Input: part model. Units: mm. Frame: model coordinates. A direction names the side the tool comes from. Coordinates: 2 decimals unless noted, no trailing zeros. Order: outer loops, then holes, each group sorted by start corner. A loop starts at its lowest first (then second) coordinate and runs counter-clockwise, first axis right, second up. Notation, with made-up numbers: (23, 22) -> (60, 22) arc R19 ccw to (60, 31) -> close; hole circle Ø7 at (-16, -31.75). An arc over 180 degrees is marked (long way). One line per item, written item: value. Start each with the question number.
from build123d import *

# Parameters (mm, degrees)
SKETCH2_W           = 10
SKETCH2_H           = 50
BOSS_EXTRUDE1_DEPTH = 10
SKETCH6_R           = 2.35
CUT_EXTRUDE3_DEPTH  = 11
SKETCH7_R           = 2.35
CUT_EXTRUDE4_DEPTH  = 11
SKETCH8_W           = 1.5
SKETCH8_H           = 21
BOSS_EXTRUDE2_DEPTH = 30


with BuildPart() as part:
    # Sketch2 → Boss-Extrude1 (new body)
    with BuildSketch(Plane.XY):
        with Locations((5, 25)):
            Rectangle(SKETCH2_W, SKETCH2_H)
    extrude(amount=BOSS_EXTRUDE1_DEPTH)

    # Sketch6 → Cut-Extrude3 (cut, through all)
    with BuildSketch(Plane.XY.offset(10)):
        with Locations((5, 27)):
            Circle(SKETCH6_R)
    extrude(amount=-CUT_EXTRUDE3_DEPTH, mode=Mode.SUBTRACT)

    # Sketch7 → Cut-Extrude4 (cut, through all)
    with BuildSketch(Plane.ZY):
        with Locations((5, 41)):
            Circle(SKETCH7_R)
        with Locations((5, 9)):
            Circle(SKETCH7_R)
    extrude(amount=-CUT_EXTRUDE4_DEPTH, mode=Mode.SUBTRACT)

    # Sketch8 → Boss-Extrude2 (add)
    with BuildSketch(Plane.ZY):
        with Locations((9.25, 26)):
            Rectangle(SKETCH8_W, SKETCH8_H)
        with Locations((0.75, 26)):
            Rectangle(SKETCH8_W, SKETCH8_H)
    extrude(amount=BOSS_EXTRUDE2_DEPTH)


solid = part.part
1) Section query D-D, the plane y = 17.5. Return the cut outline in (x, z), plus the area to 3 significant figures.
2) Pin query (flat end, axial travel): pin 1 Ø1 at (x, z) = (-8.5, 1.5) entering from -Y; pin 2 Ø1.5 at (x, z) = (-16.5, 8.5) entering from +Y. Return the tip coordinate at first contact, or that it passes through.
3) Mould query, pull axis Z, two halves, no side actions, for faces 5 (the flat face through (-6, 25, 0)), 6 (the flat face through (-15, 26, 1.5)), 7 (the flat face through (5, 50, 5)). Classes: +Z half, -Z half, draft (parallel to the pull), parting line (faces both ways), or undercut.
4) Section query A-A, the plane x = 5. Return the cut outline in (y, z), plus the area to 3 significant figures.
5) Ray query, line 1 along Z through (x, y) = (-8.5, 32); line 2 along Y through (x, z) = (5, 6); line 3 along X through (y, z) = (36.5, 2). Return the intervals inside material, ascending. Write a range as from..to.
6) Section query C-C, the plane z = 5. Return the cut outline in (x, y).
7) Section query B-B, the plane y = 27. Return the cut outline in (x, z), plus the area to 3 significant figures.
8) Access query for faces 1 (the cylindrical face through (4.93, 43.33, 4.69)), 2 (the flat face through (-15, 26, 8.5)), 3 (the flat face through (-15, 36.5, 1)), 4 (the flat face through (-15, 15.5, 1)). Directions: +Z, -Z, +X, -X, +Y, -Y. A direction counts if a zero-diameter tool reaches every point of the face in a straight line with its end or side. Return the directions, or none.
Entries:
1. outline: (-30, 0) -> (10, 0) -> (10, 10) -> (-30, 10) -> (-30, 8.5) -> (0, 8.5) -> (0, 1.5) -> (-30, 1.5) -> close
1. area: 190 mm2
2. pin 1: stops at y = 15.5
2. pin 2: stops at y = 36.5
3. face 5: -Z half
3. face 6: undercut
3. face 7: draft
4. outline: (0, 0) -> (24.65, 0) -> (24.65, 10) -> (0, 10) -> close; (29.35, 0) -> (50, 0) -> (50, 10) -> (29.35, 10) -> close; hole circle Ø4.7 at (9, 5); hole circle Ø4.7 at (41, 5)
4. area: 418 mm2
5. line 1: z = 0..1.5, 8.5..10
5. line 2: y = 0..6.87, 11.13..24.65, 29.35..38.87, 43.13..50
5. line 3: x = 0..10
6. outline: (0, 0) -> (10, 0) -> (10, 6.65) -> (0, 6.65) -> close; (0, 11.35) -> (10, 11.35) -> (10, 38.65) -> (0, 38.65) -> close; (0, 43.35) -> (10, 43.35) -> (10, 50) -> (0, 50) -> close; hole circle Ø4.7 at (5, 27)
7. outline: (-30, 0) -> (2.65, 0) -> (2.65, 10) -> (-30, 10) -> (-30, 8.5) -> (0, 8.5) -> (0, 1.5) -> (-30, 1.5) -> close; (7.35, 0) -> (10, 0) -> (10, 10) -> (7.35, 10) -> close
7. area: 143 mm2
8. face 1: +X, -X
8. face 2: -X, +Y, -Y
8. face 3: +Z, -Z, -X, +Y
8. face 4: +Z, -Z, -X, -Y
